from build123d import *

# Parameters (mm, degrees)
SKETCH1_W                       = 25
SKETCH1_H                       = 6.75
BOSS_EXTRUDE1_DEPTH             = 6.5
BOSS_EXTRUDE3_REACH             = 5.375
BOSS_EXTRUDE3_DIRECTION_2_REACH = 5.375
SKETCH4_W                       = 1
SKETCH4_H                       = 1.5
CUT_EXTRUDE1_DEPTH              = 23
BOSS_EXTRUDE4_DEPTH             = 6.5
SKETCH6_R                       = 2.55
CUT_EXTRUDE2_DEPTH              = 10
BOSS_EXTRUDE5_DEPTH             = 1.475
CUT_EXTRUDE3_DEPTH              = 3


with BuildPart() as part:
    # Sketch1 → Boss-Extrude1 (new body)
    with BuildSketch(Plane(origin=(0, 0, 0), x_dir=(1, 0, 0), z_dir=(0, 1, 0))):
        with Locations((12.5, -3.375)):
            Rectangle(SKETCH1_W, SKETCH1_H)
    extrude(amount=BOSS_EXTRUDE1_DEPTH)

    # Boss-Extrude3: up to this face of the body (flat: up to its plane)
    boss_extrude3_end = Plane(part.part.faces().sort_by_distance((12.5, 3.25, 0))[0])
    # Sketch3 → Boss-Extrude3 (add, up to the picked face)
    with BuildSketch(Plane.XY.offset(3.375), mode=Mode.PRIVATE) as boss_extrude3_sk1:
        Polygon((21.275684175, 14.155521181), (26.183820092, 15.109566157), (30, -4.522977512), (25.091864083, -5.477022488), align=None)
    boss_extrude3_tool1 = split(extrude(boss_extrude3_sk1.sketch, amount=-BOSS_EXTRUDE3_REACH, mode=Mode.PRIVATE), bisect_by=boss_extrude3_end, keep=Keep.BOTH, mode=Mode.PRIVATE)
    add(boss_extrude3_tool1.solids().sort_by_distance((25.637842, 4.816272, 3.375))[0])

    # Boss-Extrude3 direction 2: up to this face of the body (flat: up to its plane)
    boss_extrude3_direction_2_end = Plane(part.part.faces().sort_by_distance((12.5, 3.25, 6.75))[0])
    # Sketch3 → Boss-Extrude3 direction 2 (add, up to the picked face)
    with BuildSketch(Plane.XY.offset(3.375), mode=Mode.PRIVATE) as boss_extrude3_direction_2_sk1:
        Polygon((21.275684175, 14.155521181), (26.183820092, 15.109566157), (30, -4.522977512), (25.091864083, -5.477022488), align=None)
    boss_extrude3_direction_2_tool1 = split(extrude(boss_extrude3_direction_2_sk1.sketch, amount=BOSS_EXTRUDE3_DIRECTION_2_REACH, mode=Mode.PRIVATE), bisect_by=boss_extrude3_direction_2_end, keep=Keep.BOTH, mode=Mode.PRIVATE)
    add(boss_extrude3_direction_2_tool1.solids().sort_by_distance((25.637842, 4.816272, 3.375))[0])

    # Sketch4 → Cut-Extrude1 (cut)
    with BuildSketch(Plane(origin=(-1.876769127, 9.65514015, 0), x_dir=(0.981627183, 0.190808995, 0), z_dir=(-0.190808995, 0.981627183, 0))):
        with Locations((28.085790708, -3.375)):
            Rectangle(SKETCH4_W, SKETCH4_H)
    extrude(amount=-CUT_EXTRUDE1_DEPTH, mode=Mode.SUBTRACT)

    # Sketch5 → Boss-Extrude4 (add)
    with BuildSketch(Plane(origin=(0, 6.5, 0), x_dir=(1, 0, 0), z_dir=(0, 1, 0))):
        Polygon((-5.600297611, -3.375), (-2.800148806, -8.225), (2.800148806, -8.225), (5.600297611, -3.375), (2.800148806, 1.475), (-2.800148806, 1.475), align=None)
    extrude(amount=-BOSS_EXTRUDE4_DEPTH)

    # Sketch6 → Cut-Extrude2 (cut)
    with BuildSketch(Plane(origin=(0, 6.5, 0), x_dir=(1, 0, 0), z_dir=(0, 1, 0))):
        with Locations((0, -3.335615973)):
            Circle(SKETCH6_R)
    extrude(amount=-CUT_EXTRUDE2_DEPTH, mode=Mode.SUBTRACT)

    # Sketch7 → Boss-Extrude5 (add)
    with BuildSketch(Plane(origin=(0, 0, -1.475), x_dir=(-1, 0, 0), z_dir=(0, 0, -1))):
        Polygon((-2.800148806, 0), (-24.027238758, 0), (-25.091864083, -5.477022488), (-30, -4.522977512), (-26.183820092, 15.109566157), (-21.275684175, 14.155521181), (-22.763766749, 6.5), (-2.800148806, 6.5), align=None)
    extrude(amount=-BOSS_EXTRUDE5_DEPTH)

    # Sketch8 → Cut-Extrude3 (cut)
    with BuildSketch(Plane(origin=(0, 0, 0), x_dir=(-1, 0, 0), z_dir=(0, -1, 0))):
        Polygon((-4.67653718, -11.475), (4.67653718, -11.475), (9.353074361, -3.375), (4.67653718, 4.725), (-4.67653718, 4.725), (-9.353074361, -3.375), align=None)
    extrude(amount=-CUT_EXTRUDE3_DEPTH, mode=Mode.SUBTRACT)


solid = part.part
Geometry check sheet. Reference: the model listing, model coordinates, mm. A direction names the side the tool comes from. Give positions to 0.01 mm unless a question says otherwise; leave off trailing zeros. Order: outer loops, then holes, each group sorted by start corner. A loop starts at its lowest first (then second) coordinate and runs counter-clockwise, first axis right, second up.
1) Tool access check on faces 1 (the flat face through (8.39, 1.48, 5.04)), 2 (the flat face through (20, 3, 6.75)), 3 (the flat face through (27.084, 5.24, 3.386)), 4 (the flat face through (-4.2, 4.8, 5.8)). Record the directions out of +Z, -Z, +X, -X, +Y, -Y that give a thin tool (end or side, any length) a straight path to the whole face; none if there is none.
Results are:
face 1: -X, -Y
face 2: +Z, +X, +Y, -Y
face 3: +X, +Y
face 4: +Z, -X, +Y, -Y
2) Draft check along Z on faces 5 (the flat face through (15, 0, 3)), 6 (the cylindrical face through (2.432, 4.774, 2.57)), 7 (the flat face through (17, 4, -1.475)). Enter one of: released by +Z, released by -Z, zero draft, split by the parting line, or undercut.
Results are:
face 5: zero draft
face 6: undercut
face 7: released by -Z
3) Cross-section at A-A (x = 0). Record the boundary of the cut face in (y, z) (3 decimals).
Results are:
outline: (3, -1.475) - (6.5, -1.475) - (6.5, 0.786) - (3, 0.786) - close; (3, 5.886) - (6.5, 5.886) - (6.5, 8.225) - (3, 8.225) - close
4) Cross-section at D-D (y = 0.5). Record the boundary of the cut face in (x, z) (3 decimals), then the cut area to 3 significant figures.
Results are:
outline: (6.553, -1.475) - (29.024, -1.475) - (29.024, 2.625) - (28.005, 2.625) - (28.005, 4.125) - (29.024, 4.125) - (29.024, 6.75) - (7.405, 6.75) - (9.353, 3.375) - close
area: 170 mm2
5) Cross-section at B-B (z = 5.5). Record the boundary of the cut face in (x, y), then the cut area to 3 significant figures.
Results are:
outline: (-4.37, 3) - (-1.35, 3) - (-1.35, 6.5) - (-4.37, 6.5) - close; (1.35, 3) - (8.13, 3) - (8.13, 0) - (24.03, 0) - (25.09, -5.48) - (30, -4.52) - (26.18, 15.11) - (21.28, 14.16) - (22.76, 6.5) - (1.35, 6.5) - close
area: 234 mm2
6) Gauge pin test, flat ends, axial feed: pin 1 (2.5 mm diameter, centred on x = 29, y = 4.5, fed in from +Z); pin 2 (1.5 mm diameter, centred on x = 4, z = 6, fed in from -Y); pin 3 (1.4 mm diameter, centred on x = 28.5, y = 10, fed in from -Z); pin 4 (1.5 mm diameter, centred on y = 1, z = 5.5, fed in from -X). Record the tip position at first contact, or that the pin passes through.
Results are:
pin 1: stops at z = 6.75
pin 2: stops at y = 3
pin 3: passes through
pin 4: stops at x = 7.69
7) Cross-section at C-C (y = 6). Record the boundary of the cut face in (x, z) (3 decimals), then the cut area to 3 significant figures.
Results are:
outline: (-5.6, 3.375) - (-2.8, -1.475) - (27.955, -1.475) - (27.955, 2.625) - (26.936, 2.625) - (26.936, 4.125) - (27.955, 4.125) - (27.955, 6.75) - (3.652, 6.75) - (2.8, 8.225) - (-2.8, 8.225) - close; hole circle Ø5.1 at (0, 3.336)
area: 253 mm2
8) Material ranges on probe 1 along Z at (x, y) = (0, 5.1) (3 decimals); probe 2 along Y at (x, z) = (5, 0.75); probe 3 along Z at (x, y) = (25, 6) (3 decimals), recorded low to high.
Results are:
probe 1: z = -1.475 to 0.786, 5.886 to 8.225
probe 2: y = 3 to 6.5
probe 3: z = -1.475 to 6.75
